Work out the finished part from the listing and answer in its coordinate system (mm). Give positions to 0.01 mm unless a question says otherwise; leave off trailing zeros. Order: outer loops, then holes, each group sorted by start corner. A loop starts at its lowest first (then second) coordinate and runs counter-clockwise, first axis right, second up.
```python
from build123d import *


with BuildPart() as f1:
    # F0 (on Front) → F1 (revolve)
    with BuildSketch(Plane.XZ):
        with BuildLine():
            Line((-29, 31.328705), (-31, 31.328705))
            ThreePointArc((-31, 31.328705), (-32.06066, 30.889366), (-32.5, 29.828705))
            Line((-32.5, 29.828705), (-32.5, 22.828705))
            ThreePointArc((-32.5, 22.828705), (-32.06066, 21.768045), (-31, 21.328705))
            Line((-31, 21.328705), (-29, 21.328705))
            ThreePointArc((-29, 21.328705), (-27.93934, 21.768045), (-27.5, 22.828705))
            Line((-27.5, 22.828705), (-27.5, 29.828705))
            ThreePointArc((-27.5, 29.828705), (-27.93934, 30.889366), (-29, 31.328705))
        make_face()
    revolve(axis=Axis((0, 0, 21.229779), (0, 0, -1)))


solid = f1.part
```
1. Given P1, Ø2, axis at x = -22, z = 27, coming from the -Y side; P2, Ø5, axis at y = 16.5, z = 23, coming from the +X side; P3, Ø3, axis at y = 7, z = 26, coming from the -X side, each flat-ended and moving along its own axis, determine where each tip first touches the part or whether it passes through.
Findings below:
P1: stops at y = -24.8
P2: stops at x = 29.33
P3: stops at x = -32.03
2. Straight lines are drawn through the part: probe 1 along Y at (x, z) = (0, 27.25); probe 2 along Y at (x, z) = (15.5, 23.75); probe 3 along X at (y, z) = (3, 26). For each, find the intervals that lie inside material, in ascending order.
Findings below:
probe 1: y = -32.5 to -27.5, 27.5 to 32.5
probe 2: y = -28.57 to -22.72, 22.72 to 28.57
probe 3: x = -32.36 to -27.34, 27.34 to 32.36
3. The part is cut by section A-A (x = 0). Write down the section's boundary in (y, z).
Findings below:
outline: (-32.5, 22.83) arc R1.5 ccw to (-31, 21.33) - (-29, 21.33) arc R1.5 ccw to (-27.5, 22.83) - (-27.5, 29.83) arc R1.5 ccw to (-29, 31.33) - (-31, 31.33) arc R1.5 ccw to (-32.5, 29.83) - close; (27.5, 22.83) arc R1.5 ccw to (29, 21.33) - (31, 21.33) arc R1.5 ccw to (32.5, 22.83) - (32.5, 29.83) arc R1.5 ccw to (31, 31.33) - (29, 31.33) arc R1.5 ccw to (27.5, 29.83) - close
4. The mould has two halves that part along Y. Classify faces 1 (the face through (-31, 9.76, 26.28)), 2 (the face through (-21, -21, 21.329)), 3 (the face through (5.961, -26.846, 26.378)): pulls with the +Y half, pulls with the -Y half, needs draft (parallel to the pull), parting line crosses it, or undercut.
Findings below:
face 1: parting line crosses it
face 2: needs draft
face 3: undercut
5. The part is cut by section C-C (z = 28.5). Write down the section's boundary in (x, y).
Findings below:
outline: circle Ø65 at (0, 0); hole circle Ø55 at (0, 0)
